Build history of the part. All positions in model axes, mm. Face numbers are marked on the shaded views. A direction names the side the tool comes from. Coordinates: 2 decimals unless noted, no trailing zeros. Loops run counter-clockwise (first coordinate to the right, second up) from the corner with the lowest first, then second, coordinate; pieces in that order, holes last.
Item 1: Cut at A-A (x = 0). List the corners of the cut face in (y, z) (3 decimals).
Item 2: Flat gauge pins, fed straight in: pin 1 (4 mm diameter, centred on x = -3.5, y = 2.5, fed in from +Z); pin 2 (3 mm diameter, centred on x = 3, z = 14.5, fed in from -Y); pin 3 (2 mm diameter, centred on x = -4.5, z = 7, fed in from +Y). Where does each tip first touch, or does it go through?
Item 3: 3-axis set-ups, long thin cutter, end or side, ignore diameter. For the marked faces 1 and 2: which of +Z, -Z, +X, -X, +Y, -Y reach the whole face in a straight line?
Item 4: Cut at C-C (z = 23). List the corners of the cut face in (x, y) (3 decimals), and give its area (3 significant figures).
Item 5: Drill centre lines: line 1 along Z through (x, y) = (5.5, 3.5); line 2 along Z through (x, y) = (-2, 3.25); line 3 along Y through (x, z) = (-5.5, 30.5). Where is each one in solid material? Low to high.
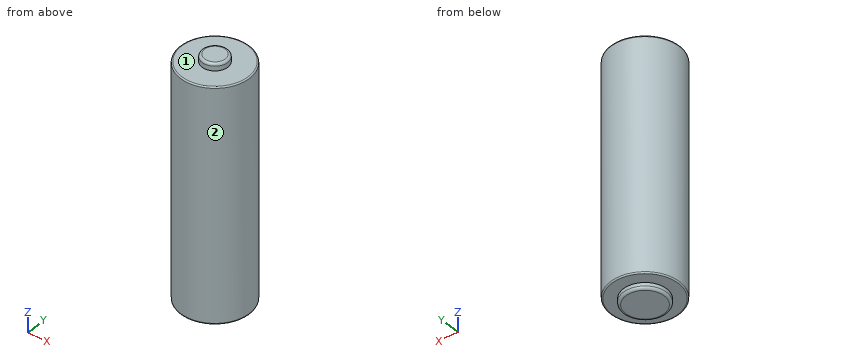
from build123d import *

# Parameters (mm, degrees)
SKETCH1_R           = 7.065
BOSS_EXTRUDE1_DEPTH = 47.5
SKETCH2_R           = 2.635
BOSS_EXTRUDE2_DEPTH = 1.45
FILLET2_R           = 0.25
SKETCH3_R           = 4.435
BOSS_EXTRUDE3_DEPTH = 1.2
FILLET1_R           = 0.5


with BuildPart() as part:
    # Sketch1 → Boss-Extrude1 (new body)
    with BuildSketch(Plane.XY):
        Circle(SKETCH1_R)
    extrude(amount=BOSS_EXTRUDE1_DEPTH)

    # Sketch2 → Boss-Extrude2 (add)
    with BuildSketch(Plane.XY.offset(47.5)):
        Circle(SKETCH2_R)
    extrude(amount=BOSS_EXTRUDE2_DEPTH)

    # Fillet2
    fillet2_edges = [part.edges().sort_by_distance(p)[0] for p in [
        (-7.065, 0, 0),
        (-7.065, 0, 47.5),
    ]]
    fillet(fillet2_edges, radius=FILLET2_R)

    # Sketch3 → Boss-Extrude3 (add)
    with BuildSketch(Plane(origin=(0, 0, 0), x_dir=(-1, 0, 0), z_dir=(0, 0, -1))):
        Circle(SKETCH3_R)
    extrude(amount=BOSS_EXTRUDE3_DEPTH)

    # Fillet1
    fillet1_edges = [part.edges().sort_by_distance(p)[0] for p in [
        (4.435, 0, -1.2),
        (-2.635, 0, 48.95),
    ]]
    fillet(fillet1_edges, radius=FILLET1_R)


solid = part.part
Filled sheet:
1. outline: (-7.065, 0.25) arc R0.25 ccw to (-6.815, 0) - (-4.435, 0) - (-4.435, -0.7) arc R0.5 ccw to (-3.935, -1.2) - (3.935, -1.2) arc R0.5 ccw to (4.435, -0.7) - (4.435, 0) - (6.815, 0) arc R0.25 ccw to (7.065, 0.25) - (7.065, 47.25) arc R0.25 ccw to (6.815, 47.5) - (2.635, 47.5) - (2.635, 48.45) arc R0.5 ccw to (2.135, 48.95) - (-2.135, 48.95) arc R0.5 ccw to (-2.635, 48.45) - (-2.635, 47.5) - (-6.815, 47.5) arc R0.25 ccw to (-7.065, 47.25) - close
2. pin 1: stops at z = 48.92
2. pin 2: stops at y = -6.9
2. pin 3: stops at y = 6.14
3. face 1: +Z
3. face 2: +Z, -Z
4. outline: circle Ø14.13 at (0, 0)
4. area: 157 mm2
5. line 1: z = 0 to 47.5
5. line 2: z = -1.2 to 47.5
5. line 3: y = -4.43 to 4.43
